Autodesk Inventor part; units mm, degrees
ref_plane "YZ Plane" through (0, 0, 0) normal (1, 0, 0) x (0, 1, 0)
ref_plane "XZ Plane" through (0, 0, 0) normal (0, 1, 0) x (-1, 0, 0)
ref_plane "XY Plane" through (0, 0, 0) normal (0, 0, 1) x (1, 0, 0)
sketch "スケッチ1" plane through (0, 0, 0) normal (0, 0, 1) x (1, 0, 0)
  circle A0 centre (13.5, 29.015) radius 1.3 construction
  circle A1 centre (-13.5, 29.015) radius 1.3 construction
  circle A2 centre (-13.5, -22.985) radius 1.3 construction
  circle A3 centre (13.5, -22.985) radius 1.3 construction
  line L0 (13.5, 29.015) -> (-13.5, 29.015) construction
  line L1 (-13.5, 29.015) -> (-13.5, -22.985) construction
  line L2 (-13.5, -22.985) -> (13.5, -22.985) construction
  line L3 (13.5, -22.985) -> (13.5, 29.015) construction
  line L4 (21.1178, -22.6697) -> (19.2418, 24.6807)
  arc A4 (19.2418, 24.6807) -> (18.3199, 28.5854) centre (8.75, 24.265) ccw
  line L5 (0, 0) -> (0, -35.9566) construction
  circle A5 centre (-12.061, 67.9318) radius 5
  line L6 (-16.75, -30.235) -> (-15.5, -30.235)
  arc A6 (-15.5, -30.235) -> (-12.5, -30.235) centre (-14, -28.235) ccw
  line L7 (-12.5, -30.235) -> (-6.1, -30.235)
  line L8 (-6.1, -30.235) -> (-6.1, -27.6492)
  arc A7 (-4.6858, -26.235) -> (-6.1, -27.6492) centre (-5.3929, -26.9421) ccw
  line L9 (-4.6858, -26.235) -> (4.6858, -26.235)
  arc A8 (6.1, -27.6492) -> (4.6858, -26.235) centre (5.3929, -26.9421) ccw
  line L10 (6.1, -27.6492) -> (6.1, -30.235)
  line L11 (6.1, -30.235) -> (12.5, -30.235)
  arc A9 (12.5, -30.235) -> (15.5, -30.235) centre (14, -28.235) ccw
  line L12 (15.5, -30.235) -> (16.75, -30.235)
  arc A10 (-11.25, -10.8278) -> (11.25, -6.4392) centre (0.8, -12.735) ccw construction
  circle A11 centre (0.8, -12.735) radius 12.2
  circle A12 centre (-12.061, 67.9318) radius 5 construction
  circle A13 centre (8.75, 24.265) radius 3 construction
  line L13 (-11.25, 1.4772) -> (-11.25, 21.265)
  arc A14 (-6.25, 26.265) -> (-11.25, 21.265) centre (-6.25, 21.265) ccw
  line L14 (-6.25, 26.265) -> (1.25, 26.265)
  line L15 (11.25, 16.765) -> (11.25, 2.5355)
  arc A15 (2.25, 24.265) -> (8.75, 17.765) centre (8.75, 24.265) ccw
  line L16 (8.75, 17.765) -> (10.25, 17.765)
  line L17 (2.25, 24.265) -> (2.25, 25.265)
  arc A16 (11.25, 16.765) -> (10.25, 17.765) centre (10.25, 16.765) ccw
  arc A17 (2.25, 25.265) -> (1.25, 26.265) centre (1.25, 25.265) ccw
  arc A18 (8.9915, 1.2414) -> (-8.8559, 0.2728) centre (0.8, -12.735) ccw
  arc A19 (8.9915, 1.2414) -> (11.25, 2.5355) centre (9.75, 2.5355) ccw
  arc A20 (-11.25, 1.4772) -> (-8.8559, 0.2728) centre (-9.75, 1.4772) ccw
  line L18 (18.3199, 28.5854) -> (-1.5796, 72.6637)
  arc A21 (-1.5796, 72.6637) -> (-23.0621, 64.5812) centre (-12.061, 67.9318) ccw
  line L19 (-18.25, -25.6185) -> (-16.75, -30.235)
  line L20 (16.75, -30.235) -> (21.1178, -22.6697)
  line L21 (16.0414, 27.5568) -> (-3.8582, 71.635) construction
  arc A22 (16.7437, 24.5817) -> (16.0414, 27.5568) centre (8.75, 24.265) ccw construction
  line L22 (18.7764, -26.7219) -> (16.7437, 24.5817) construction
  arc A23 (-15.75, 32.265) -> (-20.6705, 65.3096) centre (-129.1686, 32.265) ccw construction
  line L23 (-15.75, 32.265) -> (-15.75, -31.3287) construction
  line L24 (-18.25, -25.6185) -> (-18.25, 32.265)
  arc A24 (-18.25, 32.265) -> (-23.0621, 64.5812) centre (-129.1686, 32.265) ccw
  point P0 (0, -56.485)
  point P1 (11.25, -0.3561)
  point P2 (-11.25, -1.9074)
  dimension "d3" = 10
  dimension "d22" = 3.5
  dimension "d23" = 1
  dimension "d24" = 1.5
  dimension "d25" = 4
  dimension "d35" = 11.5
  dimension "d37" = 18
  dimension "d38" = 30
extrude "押し出し1" add sketch "スケッチ1" against normal blind 2
hole "穴1" at (-13.5, 29.015, 0) at (-13.5, -22.985, 0) at (13.5, -22.985, 0) at (13.5, 29.015, 0) direction (0, 0, -1) diameter 2.9 end through all countersink diameter 5.5 countersink angle 90
hole "穴2" at (14, -28.235, 0) at (-14, -28.235, 0) direction (0, 0, -1) diameter 2 end through all
hole "穴3" at (8.75, 24.265, 0) direction (0, 0, -1) diameter 6 end through all counterbore diameter 7.3 counterbore depth 0.65
properties part number "UPPER_LEG_MIDDLE_FRAME"
Geometry: final body of the model. Coordinates: model frame, mm. A direction names the side the tool comes from. Coordinates: 2 decimals unless noted, no trailing zeros. Order: outer loops, then holes, each group sorted by start corner. A loop starts at its lowest first (then second) coordinate and runs counter-clockwise, first axis right, second up. Notation, with made-up numbers: (-0.75, -14.75) -> (31.25, -14.75) arc R25 cw to (31.25, 4.25) -> close; hole circle Ø9 at (25.25, -25.5). An arc over 180 degrees is marked (long way). Write item = value, one per line.
(1) Pin query (flat end, axial travel): pin 1 Ø1.1 at (y, z) = (24.5, -0.5) entering from -X; pin 2 Ø1 at (x, z) = (0, -1.5) entering from -Y (3 decimals); pin 3 Ø1.5 at (x, y) = (8, 26.5) entering from +Z. Return the tip coordinate at first contact, or that it passes through.
Solved:
pin_1 = -18.25
pin_2 = -26.235
pin_3 = -0.65
(2) Cut plane B-B on x = -0.5. Return loops of the section in (y, z) (3 decimals).
Solved:
outline = (-26.235, -2) -> (-24.866, -2) -> (-24.866, 0) -> (-26.235, 0) -> close; (-0.604, -2) -> (3.413, -2) -> (3.413, 0) -> (-0.604, 0) -> close; (26.265, -2) -> (70.272, -2) -> (70.272, 0) -> (26.265, 0) -> close
(3) Line query: line 1 (Y direction, x = 13.5, z = -1.6) (3 decimals); line 2 (Y direction, x = -1, z = -1.05) (3 decimals); line 3 (Y direction, x = -13.5, z = -1.65) (3 decimals). Output: solid intervals per line, ascending.
Solved:
line_1 = -30.684 to -29.101, -27.369 to -24.435, -21.535 to 27.565, 30.465 to 39.262
line_2 = -26.235 to -24.801, -0.669 to 3.365, 26.265 to 71.38
line_3 = -30.684 to -29.101, -27.369 to -24.435, -21.535 to 27.565, 30.465 to 63.143, 72.72 to 79.341
(4) Cut plane A-A on y = -14. Return loops of the section in (x, z).
Solved:
outline = (-18.25, -2) -> (-11.33, -2) -> (-11.33, 0) -> (-18.25, 0) -> close; (12.93, -2) -> (20.77, -2) -> (20.77, 0) -> (12.93, 0) -> close
(5) Access query for faces 4 (the flat face through (12, 25, -0.65)), 5 (the flat face through (-6.1, -29, -1)), 6 (the flat face through (-3, 26.265, -1)). Directions: +Z, -Z, +X, -X, +Y, -Y. A direction counts if a zero-diameter tool reaches every point of the face in a straight line with its end or side. Return the directions, or none.
Solved:
face_4 = +Z
face_5 = +Z, -Z, -Y
face_6 = +Z, -Z
(6) Pull-direction query (X, two-part tool) for faces 1 (the cylindrical face through (4.104, 19.72, -0.986)), 2 (the cylindrical face through (-15.88, 78.78, -0.99)), 3 (the flat face through (3, 25, -2)); classes: pulls with the +X half, pulls with the -X half, needs draft (parallel to the pull), parting line crosses it, or undercut.
Solved:
face_1 = undercut
face_2 = parting line crosses it
face_3 = needs draft
(7) Cut plane C-C on y = 8.5. Return loops of the section in (x, z).
Solved:
outline = (-18.25, -2) -> (-11.25, -2) -> (-11.25, 0) -> (-18.25, 0) -> close; (11.25, -2) -> (19.88, -2) -> (19.88, 0) -> (11.25, 0) -> close
(8) Cut plane D-D on y = 37. Return loops of the section in (x, z), plus the area to 3 significant figures.
Solved:
outline = (-18.35, -2) -> (14.52, -2) -> (14.52, 0) -> (-18.35, 0) -> close
area = 65.7 mm²
